from build123d import *
from build123d.topology import SkipClean

# Parameters (mm, degrees)
SKETCH1_W                  = 9
SKETCH1_H                  = 9
BOSS_EXTRUDE1_DEPTH        = 3
HOLE1_AT_2_COUNT           = 2
HOLE1_AT_2_PITCH           = 6
HOLE1_AT_3_COUNT           = 2
HOLE1_AT_3_PITCH           = 6
BOSS_EXTRUDE2_DEPTH        = 2.2
HOLE2_D                    = 4
HOLE2_DEPTH                = 2.2
HOLE2_CBORE_D              = 5
HOLE2_CBORE_DEPTH          = 0.8
MIRROR2_COPY_3_SKETCH_W    = 9
MIRROR2_COPY_3_SKETCH_H    = 9
MIRROR2_COPY_3_DEPTH       = 3
MIRROR2_COPY_5_DEPTH       = 2.2
MIRROR2_COPY_6_D           = 4
MIRROR2_COPY_6_DEPTH       = 2.2
MIRROR2_COPY_6_CBORE_D     = 5
MIRROR2_COPY_6_CBORE_DEPTH = 0.8


with BuildPart() as part:
    # Sketch1 → Boss-Extrude1 (new body)
    with BuildSketch(Plane(origin=(0, 0, 0), x_dir=(1, 0, 0), z_dir=(0, 1, 0))):
        with Locations((4.5, 0)):
            Rectangle(SKETCH1_W, SKETCH1_H)
    boss_extrude1 = extrude(amount=-BOSS_EXTRUDE1_DEPTH)

    # Sketch5 → Hole1 (revolve, cut)
    with BuildSketch(Plane(origin=(9, 0, 4.5), x_dir=(0, 0, 1), z_dir=(1, 0, 0))):
        Polygon((0, 0), (0, 4.201721238), (2, 3), (2, 0.8), (2.5, 0.8), (2.5, 0), align=None)
    hole1 = revolve(axis=Axis((9, 11.310875039, 4.5), (0, -1, 0)), mode=Mode.SUBTRACT)

    # Hole1 at 2: Hole1 ×2
    with Locations(*[(0, 0, -i * HOLE1_AT_2_PITCH) for i in range(1, HOLE1_AT_2_COUNT)]):
        add(hole1, mode=Mode.SUBTRACT)

    # Hole1 at 3: Hole1 ×2
    with Locations(*[(-i * HOLE1_AT_3_PITCH, 0, 0) for i in range(1, HOLE1_AT_3_COUNT)]):
        add(hole1, mode=Mode.SUBTRACT)

    # Sketch6 → Boss-Extrude2 (add)
    with BuildSketch(Plane(origin=(0, 0, 0), x_dir=(0, 0, -1), z_dir=(1, 0, 0))):
        with BuildLine():
            Line((4.5, 0), (-1.5, 0))
            ThreePointArc((-1.5, 0), (1.5, 3), (4.5, 0))
        make_face()
    boss_extrude2 = extrude(amount=BOSS_EXTRUDE2_DEPTH)

    # Hole2
    with Locations(Plane.ZY):
        with Locations((-1.5, 0)):
            hole2 = CounterBoreHole(HOLE2_D / 2, HOLE2_CBORE_D / 2, HOLE2_CBORE_DEPTH, depth=HOLE2_DEPTH)

    # Mirror1: Boss-Extrude1, Hole1, Boss-Extrude2, Hole2 across plane
    add(boss_extrude1.mirror(Plane.XY.offset(4.5)))
    add(hole1.mirror(Plane.XY.offset(4.5)), mode=Mode.SUBTRACT)
    add(boss_extrude2.mirror(Plane.XY.offset(4.5)))
    add(hole2.mirror(Plane.XY.offset(4.5)), mode=Mode.SUBTRACT)

    # Mirror1 copy 1 sketch → Mirror1 copy 1 (revolve, cut)
    with BuildSketch(Plane(origin=(9, 0, 10.5), x_dir=(0, 0, -1), z_dir=(1, 0, 0))):
        Polygon((0, 0), (0, -4.201721238), (2, -3), (2, -0.8), (2.5, -0.8), (2.5, 0), align=None)
    revolve(axis=Axis((9, 11.310875039, 10.5), (0, 1, 0)), mode=Mode.SUBTRACT)

    # Mirror1 copy 2 sketch → Mirror1 copy 2 (revolve, cut)
    with BuildSketch(Plane(origin=(3, 0, 4.5), x_dir=(0, 0, -1), z_dir=(1, 0, 0))):
        Polygon((0, 0), (0, -4.201721238), (2, -3), (2, -0.8), (2.5, -0.8), (2.5, 0), align=None)
    revolve(axis=Axis((3, 11.310875039, 4.5), (0, 1, 0)), mode=Mode.SUBTRACT)

    # Mirror2: Boss-Extrude1, Hole1, Boss-Extrude2, Hole2 across plane
    with SkipClean():  # the faces are left unmerged after this step: merging them gives an invalid solid
        add(boss_extrude1.mirror(Plane(origin=(9, 0, 0), x_dir=(0, 0, 1), z_dir=(1, 0, 0))))
        add(hole1.mirror(Plane(origin=(9, 0, 0), x_dir=(0, 0, 1), z_dir=(1, 0, 0))), mode=Mode.SUBTRACT)
        add(boss_extrude2.mirror(Plane(origin=(9, 0, 0), x_dir=(0, 0, 1), z_dir=(1, 0, 0))))
        add(hole2.mirror(Plane(origin=(9, 0, 0), x_dir=(0, 0, 1), z_dir=(1, 0, 0))), mode=Mode.SUBTRACT)

    # Mirror2 copy 1 sketch → Mirror2 copy 1 (revolve, cut)
    with SkipClean():  # the faces are left unmerged after this step: merging them gives an invalid solid
        with BuildSketch(Plane(origin=(9, 0, -1.5), x_dir=(0, 0, 1), z_dir=(-1, 0, 0))):
            Polygon((0, 0), (0, -4.201721238), (2, -3), (2, -0.8), (2.5, -0.8), (2.5, 0), align=None)
        revolve(axis=Axis((9, 11.310875039, -1.5), (0, 1, 0)), mode=Mode.SUBTRACT)
    add(part.part.scale(1), mode=Mode.REPLACE)  # the faces are merged on a copy

    # Mirror2 copy 2 sketch → Mirror2 copy 2 (revolve, cut)
    with BuildSketch(Plane(origin=(15, 0, 4.5), x_dir=(0, 0, 1), z_dir=(-1, 0, 0))):
        Polygon((0, 0), (0, -4.201721238), (2, -3), (2, -0.8), (2.5, -0.8), (2.5, 0), align=None)
    revolve(axis=Axis((15, 11.310875039, 4.5), (0, 1, 0)), mode=Mode.SUBTRACT)

    # Mirror2 copy 3 sketch → Mirror2 copy 3 (add)
    with BuildSketch(Plane(origin=(18, 0, 9), x_dir=(-1, 0, 0), z_dir=(0, 1, 0))):
        with Locations((4.5, 0)):
            Rectangle(MIRROR2_COPY_3_SKETCH_W, MIRROR2_COPY_3_SKETCH_H)
    extrude(amount=-MIRROR2_COPY_3_DEPTH)

    # Mirror2 copy 4 sketch → Mirror2 copy 4 (revolve, cut)
    with BuildSketch(Plane(origin=(9, 0, 4.5), x_dir=(0, 0, -1), z_dir=(-1, 0, 0))):
        Polygon((0, 0), (0, 4.201721238), (2, 3), (2, 0.8), (2.5, 0.8), (2.5, 0), align=None)
    revolve(axis=Axis((9, 11.310875039, 4.5), (0, -1, 0)), mode=Mode.SUBTRACT)

    # Mirror2 copy 5 sketch → Mirror2 copy 5 (add)
    with BuildSketch(Plane(origin=(18, 0, 9), x_dir=(0, 0, 1), z_dir=(-1, 0, 0))):
        with BuildLine():
            Line((4.5, 0), (-1.5, 0))
            ThreePointArc((-1.5, 0), (1.5, 3), (4.5, 0))
        make_face()
    extrude(amount=MIRROR2_COPY_5_DEPTH)

    # Mirror2 copy 6
    with Locations(Plane(origin=(18, 0, 9), x_dir=(0, 0, -1), z_dir=(1, 0, 0))):
        with Locations((-1.5, 0)):
            CounterBoreHole(MIRROR2_COPY_6_D / 2, MIRROR2_COPY_6_CBORE_D / 2, MIRROR2_COPY_6_CBORE_DEPTH, depth=MIRROR2_COPY_6_DEPTH)

    # Mirror2 copy 7 sketch → Mirror2 copy 7 (revolve, cut)
    with BuildSketch(Plane(origin=(9, 0, 10.5), x_dir=(0, 0, -1), z_dir=(-1, 0, 0))):
        Polygon((0, 0), (0, 4.201721238), (2, 3), (2, 0.8), (2.5, 0.8), (2.5, 0), align=None)
    revolve(axis=Axis((9, 11.310875039, 10.5), (0, -1, 0)), mode=Mode.SUBTRACT)

    # Mirror2 copy 8 sketch → Mirror2 copy 8 (revolve, cut)
    with SkipClean():  # the faces are left unmerged after this step: merging them gives an invalid solid
        with BuildSketch(Plane(origin=(15, 0, 4.5), x_dir=(0, 0, -1), z_dir=(-1, 0, 0))):
            Polygon((0, 0), (0, 4.201721238), (2, 3), (2, 0.8), (2.5, 0.8), (2.5, 0), align=None)
        revolve(axis=Axis((15, 11.310875039, 4.5), (0, -1, 0)), mode=Mode.SUBTRACT)
    add(part.part.scale(1), mode=Mode.REPLACE)  # the faces are merged on a copy


solid = part.part
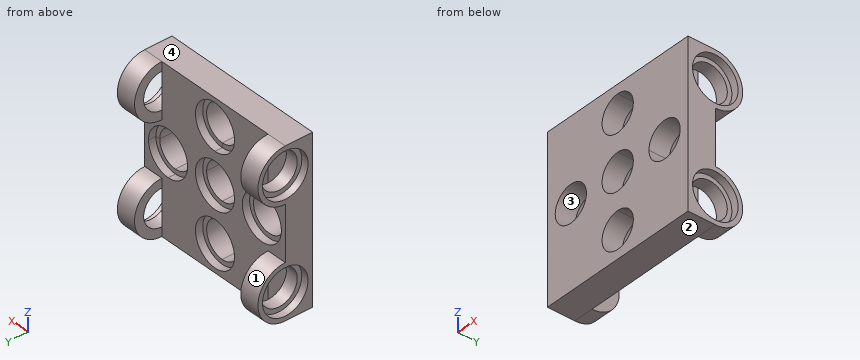
Can you work these out from the model? Positions are in its coordinate system, mm. Face numbers are marked on the shaded views. Give positions to 0.01 mm unless a question says otherwise; leave off trailing zeros. Loops run counter-clockwise (first coordinate to the right, second up) from the corner with the lowest first, then second, coordinate; pieces in that order, holes last. Notation, with made-up numbers: (44.25, -10.5) -> (71.25, -10.5) arc R12 cw to (71.25, 6.5) -> close; hole circle Ø3 at (3.5, 37.5). An arc over 180 degrees is marked (long way). Return JSON: item names as keys, results as strings.
Q1. For pin 1 Ø1.5 at (y, z) = (-0.5, 9) entering from +X; pin 2 Ø5.5 at (x, z) = (12.5, 5.5) entering from +Y; pin 3 Ø2 at (x, z) = (14, 5.5) entering from +Y; pin 4 Ø3 at (x, z) = (3, 4.5) entering from +Y, each with a flat end and sliding along its axis, tell me the tip position at first contact or that it passes through.
Checks:
{"pin 1": "stops at x = 17.2", "pin 2": "stops at y = 0", "pin 3": "stops at y = -0.8", "pin 4": "passes through"}
Q2. We'd pull the mould along Z, two halves only. Please class the marked faces 1, 2, 3 and 4: released by +Z, released by -Z, zero draft, split by the parting line, or undercut.
Checks:
{"face 1": "undercut", "face 2": "released by -Z", "face 3": "undercut", "face 4": "released by +Z"}
Q3. I want a section at A-A, the plane z = -1.5. Count the separate pieces of the cut face and the enclosed holes in it, then the cut area to 3 significant figures.
Checks:
{"separate pieces": "4", "enclosed holes": "0", "area": "35.2 mm2"}
Q4. I want a section at C-C, the plane x = 3.5. List the corners of the cut face in (y, z) for me, then the cut area to 3 significant figures.
Checks:
{"outline": "(-3, -4.5) -> (0, -4.5) -> (0, 2.05) -> (-0.8, 2.05) -> (-0.8, 2.56) -> (-3, 2.56) -> close; (-3, 6.44) -> (-0.8, 6.44) -> (-0.8, 6.95) -> (0, 6.95) -> (0, 13.5) -> (-3, 13.5) -> close", "area": "41.6 mm2"}
Q5. I want a section at D-D, the plane z = 5. List the corners of the cut face in (x, y) for me.
Checks:
{"outline": "(0, -3) -> (1.06, -3) -> (1.06, -0.8) -> (0.55, -0.8) -> (0.55, 0) -> (0, 0) -> close; (4.94, -3) -> (7.06, -3) -> (7.06, -0.8) -> (6.55, -0.8) -> (6.55, 0) -> (5.45, 0) -> (5.45, -0.8) -> (4.94, -0.8) -> close; (10.94, -3) -> (13.06, -3) -> (13.06, -0.8) -> (12.55, -0.8) -> (12.55, 0) -> (11.45, 0) -> (11.45, -0.8) -> (10.94, -0.8) -> close; (16.94, -3) -> (18, -3) -> (18, 0) -> (17.45, 0) -> (17.45, -0.8) -> (16.94, -0.8) -> close"}
Q6. I need wall thicknesses on probe 1 along Z at (x, y) = (9, -0.6); probe 2 along X at (y, z) = (-1.45, 4.5); probe 3 along Y at (x, z) = (16.75, 10.5). Which ranges of each line are inside material? Lowest first, please.
Checks:
{"probe 1": "z = -4.5 to -4, 1 to 2, 7 to 8, 13 to 13.5", "probe 2": "x = 0 to 1, 5 to 7, 11 to 13, 17 to 18", "probe 3": "y = -3 to -2, 2 to 3"}
Q7. I want a section at B-B, the plane x = 10.25. List the corners of the cut face in (y, z) for me, then the cut area to 3 significant figures.
Checks:
{"outline": "(-3, -4.5) -> (0, -4.5) -> (0, -3.67) -> (-0.8, -3.67) -> (-0.8, -3.06) -> (-3, -3.06) -> close; (-3, 0.06) -> (-0.8, 0.06) -> (-0.8, 0.67) -> (0, 0.67) -> (0, 2.33) -> (-0.8, 2.33) -> (-0.8, 2.94) -> (-3, 2.94) -> close; (-3, 6.06) -> (-0.8, 6.06) -> (-0.8, 6.67) -> (0, 6.67) -> (0, 8.33) -> (-0.8, 8.33) -> (-0.8, 8.94) -> (-3, 8.94) -> close; (-3, 12.06) -> (-0.8, 12.06) -> (-0.8, 12.67) -> (0, 12.67) -> (0, 13.5) -> (-3, 13.5) -> close", "area": "23.0 mm2"}
